Could you check a few things on this model? Use its own coordinates, in mm. Give positions to 0.01 mm unless a question says otherwise; leave off trailing zeros. Order: outer loops, then holes, each group sorted by start corner. A loop starts at its lowest first (then second) coordinate and runs counter-clockwise, first axis right, second up. Notation, with made-up numbers: (1, 9.5) - (58, 9.5) arc R29 ccw to (58, 33.5) - close; hole circle Ø3 at (-5, -1). An arc over 180 degrees is marked (long way). One line per question, with ' | ' between items. Start each with the question number.
1. Imagine slicing it at D-D (y = 14.25). Please give me the cut outline in (x, z), and give its area (3 significant figures).
2. Imagine slicing it at C-C (x = 40.5). Please give me the cut outline in (y, z).
3. Imagine slicing it at B-B (y = 0.5). Please give me the cut outline in (x, z), and give its area (3 significant figures).
4. If we mould it in two halves opening along Y, with no side actions, what happens to faces 1 (the flat face through (-1, 0, 0)), 2 (the cylindrical face through (40.604, -13.457, -2.028)), 3 (the flat face through (-1, 17.75, -2)), 4 (the cylindrical face through (-40.396, -13.457, -2.028))? For each: released by +Y, released by -Y, zero draft, split by the parting line, or undercut.
5. I need wall thicknesses on probe 1 along Y at (x, z) = (-40.5, -1.85); probe 2 along Y at (x, z) = (12.55, -1.7); probe 3 along X at (y, z) = (2.5, -3.55). Which ranges of each line are inside material? Lowest first, please. Write a range as from..to.
6. For P1, Ø15.5, axis at x = 12.55, y = 7.75, coming from the -Z side; P2, Ø19.5, axis at x = -12.55, y = 7.62, coming from the -Z side, each with a flat end and sliding along its axis, tell me the tip position at first contact or that it passes through.
7. Imagine slicing it at A-A (x = 12.55). Please give me the cut outline in (y, z).
```python
from build123d import *

# Parameters (mm, degrees)
SKETCH1_W             = 85.5
SKETCH1_H             = 35.5
BOSS_EXTRUDE1_DEPTH   = 4
M2_TAPPED_HOLE1_D     = 1.6
M2_TAPPED_HOLE1_DEPTH = 6
M2_TAPPED_HOLE1_TIP   = 0.480688495
SKETCH4_R             = 8.5
CUT_EXTRUDE1_DEPTH    = 10


with BuildPart() as part:
    # Sketch1 → Boss-Extrude1 (new body)
    with BuildSketch(Plane.XY):
        Rectangle(SKETCH1_W, SKETCH1_H)
    extrude(amount=-BOSS_EXTRUDE1_DEPTH)

    # M2 Tapped Hole1
    with Locations(Plane.XY):
        with Locations((40.5, 14.25), (-40.5, 14.25), (40.5, -14.25), (-40.5, -14.25)):
            Hole(M2_TAPPED_HOLE1_D / 2, depth=M2_TAPPED_HOLE1_DEPTH)
            with Locations((0, 0, -(M2_TAPPED_HOLE1_DEPTH + M2_TAPPED_HOLE1_TIP / 2))):  # 118° drill point
                Cone(0, M2_TAPPED_HOLE1_D / 2, M2_TAPPED_HOLE1_TIP, mode=Mode.SUBTRACT)

    # Sketch4 → Cut-Extrude1 (cut)
    with BuildSketch(Plane.XY):
        with Locations((12.55, 7.75)):
            Circle(SKETCH4_R)
        with Locations((-12.55, 7.61724702)):
            Circle(SKETCH4_R)
    extrude(amount=-CUT_EXTRUDE1_DEPTH, mode=Mode.SUBTRACT)


solid = part.part
```
Results found:
1) outline: (-42.75, -4) - (-41.3, -4) - (-41.3, 0) - (-42.75, 0) - close; (-39.7, -4) - (-17.87, -4) - (-17.87, 0) - (-39.7, 0) - close; (-7.23, -4) - (7.07, -4) - (7.07, 0) - (-7.23, 0) - close; (18.03, -4) - (39.7, -4) - (39.7, 0) - (18.03, 0) - close; (41.3, -4) - (42.75, -4) - (42.75, 0) - (41.3, 0) - close | area: 243 mm2
2) outline: (-17.75, -4) - (-15.05, -4) - (-15.05, 0) - (-17.75, 0) - close; (-13.45, -4) - (13.45, -4) - (13.45, 0) - (-13.45, 0) - close; (15.05, -4) - (17.75, -4) - (17.75, 0) - (15.05, 0) - close
3) outline: (-42.75, -4) - (-17.2, -4) - (-17.2, 0) - (-42.75, 0) - close; (-7.9, -4) - (8.11, -4) - (8.11, 0) - (-7.9, 0) - close; (16.99, -4) - (42.75, -4) - (42.75, 0) - (16.99, 0) - close | area: 269 mm2
4) face 1: zero draft | face 2: undercut | face 3: released by +Y | face 4: undercut
5) probe 1: y = -17.75..-15.05, -13.45..13.45, 15.05..17.75 | probe 2: y = -17.75..-0.75, 16.25..17.75 | probe 3: x = -42.75..-19.34, -5.76..5.87, 19.23..42.75
6) P1: passes through | P2: stops at z = -4
7) outline: (-17.75, -4) - (-0.75, -4) - (-0.75, 0) - (-17.75, 0) - close; (16.25, -4) - (17.75, -4) - (17.75, 0) - (16.25, 0) - close
